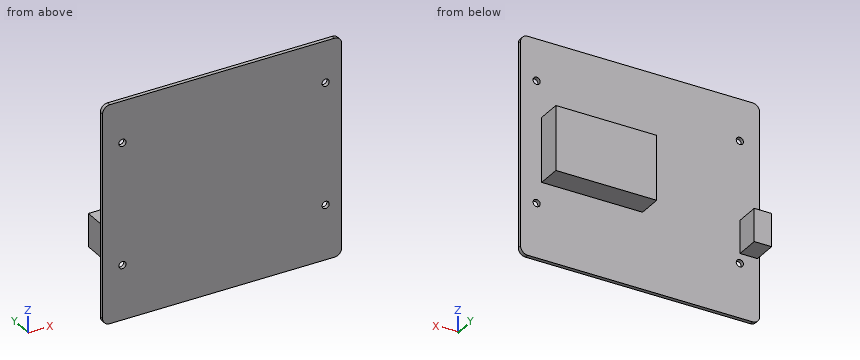
```python
from build123d import *

# Parameters (mm, degrees)
SKETCH_1_R      = 1.5
EXTRUDE_1_DEPTH = 1.6
SKETCH_2_W      = 42.186521795
SKETCH_2_H      = 26.994351744
SKETCH_2_W_2    = 7.282197215
SKETCH_2_H_2    = 13.811063683
EXTRUDE_2_DEPTH = 10


with BuildPart() as part:
    # 草图1 → 凸台-拉伸1 (new body)
    with BuildSketch(Plane(origin=(0, 0, 0), x_dir=(1, 0, 0), z_dir=(0, 1, 0))):
        with BuildLine():
            Line((-47, 45.5), (47, 45.5))
            ThreePointArc((47, 45.5), (49.121320344, 44.621320344), (50, 42.5))
            Line((50, 42.5), (50, -42.5))
            ThreePointArc((50, -42.5), (49.121320344, -44.621320344), (47, -45.5))
            Line((47, -45.5), (-47, -45.5))
            ThreePointArc((-47, -45.5), (-49.121320344, -44.621320344), (-50, -42.5))
            Line((-50, -42.5), (-50, 42.5))
            ThreePointArc((-50, 42.5), (-49.121320344, 44.621320344), (-47, 45.5))
        make_face()
        with Locations(Location((-41.7, 22.7, 0), (0, 0, 270))):
            Circle(SKETCH_1_R, mode=Mode.SUBTRACT)
        with Locations(Location((43.3, 22.7, 0), (0, 0, 270))):
            Circle(SKETCH_1_R, mode=Mode.SUBTRACT)
        with Locations(Location((43.3, -28.1, 0), (0, 0, 270))):
            Circle(SKETCH_1_R, mode=Mode.SUBTRACT)
        with Locations(Location((-41.7, -28.1, 0), (0, 0, 270))):
            Circle(SKETCH_1_R, mode=Mode.SUBTRACT)
    extrude(amount=EXTRUDE_1_DEPTH)

    # 草图2 → 凸台-拉伸2 (add)
    with BuildSketch(Plane(origin=(0, 1.6, 0), x_dir=(1, 0, 0), z_dir=(0, 1, 0))):
        with Locations((20.088819902, 0)):
            Rectangle(SKETCH_2_W, SKETCH_2_H)
        with Locations((-45.45095503, 11.739404131)):
            Rectangle(SKETCH_2_W_2, SKETCH_2_H_2)
    extrude(amount=EXTRUDE_2_DEPTH)


solid = part.part
```
Can you work these out from the model? Positions are in its coordinate system, mm. Coordinates: 2 decimals unless noted, no trailing zeros. Write each loop counter-clockwise with the first axis right and the second up, starting at its lowest first coordinate (ties: lowest second). Pieces come first, ordered by that corner, then holes. Notation, with made-up numbers: (66, -29) - (105, -29) arc R24 cw to (105, 9) - close; hole circle Ø2 at (32, 46). An arc over 180 degrees is marked (long way). Return JSON: item names as keys, results as strings.
Q1. If we section it at B-B (y = 10): Please give me the cut outline in (x, z).
Computed values:
{"outline": "(-49.09, -18.64) - (-41.81, -18.64) - (-41.81, -4.83) - (-49.09, -4.83) - close; (-1, -13.5) - (41.18, -13.5) - (41.18, 13.5) - (-1, 13.5) - close"}
Q2. If we section it at C-C (x = 43.3): Please give me the cut outline in (y, z), then the cut area to 3 significant figures.
Computed values:
{"outline": "(0, -45.5) - (1.6, -45.5) - (1.6, -24.2) - (0, -24.2) - close; (0, -21.2) - (1.6, -21.2) - (1.6, 26.6) - (0, 26.6) - close; (0, 29.6) - (1.6, 29.6) - (1.6, 45.5) - (0, 45.5) - close", "area": "136 mm2"}
Q3. If we section it at D-D (x = 32.5): Please give me the cut outline in (y, z), then the cut area to 3 significant figures.
Computed values:
{"outline": "(0, -45.5) - (1.6, -45.5) - (1.6, -13.5) - (11.6, -13.5) - (11.6, 13.5) - (1.6, 13.5) - (1.6, 45.5) - (0, 45.5) - close", "area": "416 mm2"}
Q4. Please list where these lines run through material, in increasing order: L1, parallel to X at y = 1.2, z = 28.1; L2, parallel to Y at x = 38, z = 15; L3, parallel to Z at x = 29, y = 9. Write a range as from..to.
Computed values:
{"L1": "x = -50..-43.2, -40.2..41.8, 44.8..50", "L2": "y = 0..1.6", "L3": "z = -13.5..13.5"}
Q5. I'm going to push flat-ended pins straight in: pin 1 Ø6 at (x, y) = (-46, 4.5) entering from +Z; pin 2 Ø4 at (x, z) = (43.3, -22.7) entering from +Y; pin 3 Ø4 at (y, z) = (4, -9.5) entering from -X; pin 4 Ø3 at (y, z) = (8, 0) entering from -X. Where does each tip first touch, or does it pass through?
Computed values:
{"pin 1": "stops at z = 45.5", "pin 2": "stops at y = 1.6", "pin 3": "stops at x = -49.09", "pin 4": "stops at x = -1"}
Q6. If we section it at A-A (z = -22.7): Please give me the cut outline in (x, y), then the cut area to 3 significant figures.
Computed values:
{"outline": "(-50, 0) - (-43.2, 0) - (-43.2, 1.6) - (-50, 1.6) - close; (-40.2, 0) - (41.8, 0) - (41.8, 1.6) - (-40.2, 1.6) - close; (44.8, 0) - (50, 0) - (50, 1.6) - (44.8, 1.6) - close", "area": "150 mm2"}
